Autodesk Inventor part; units mm, degrees
ref_plane "YZ Plane" through (0, 0, 0) normal (1, 0, 0) x (0, 1, 0)
ref_plane "XZ Plane" through (0, 0, 0) normal (0, 1, 0) x (-1, 0, 0)
ref_plane "XY Plane" through (0, 0, 0) normal (0, 0, 1) x (1, 0, 0)
sketch "Sketch1" plane through (0, 0, 0) normal (0, 1, 0) x (-1, 0, 0)
  line L0 (78.74, -3.175) -> (78.74, -41.275)
  line L1 (0, -41.275) -> (0, -3.175)
  line L2 (74.295, -4.445) -> (4.445, -4.445)
  line L3 (4.445, -4.445) -> (4.445, -40.005)
  line L4 (4.445, -40.005) -> (74.295, -40.005)
  line L5 (74.295, -40.005) -> (74.295, -4.445)
  line L6 (78.74, -3.175) -> (75.565, 0)
  line L7 (78.74, -41.275) -> (75.565, -44.45)
  line L8 (3.175, -44.45) -> (0, -41.275)
  line L9 (0, -3.175) -> (3.175, 0)
  line L10 (62.865, 0) -> (62.865, 12.7)
  line L11 (62.865, 12.7) -> (75.565, 12.7)
  line L12 (75.565, 12.7) -> (75.565, 0)
  line L13 (62.865, -44.45) -> (62.865, -57.15)
  line L14 (62.865, -57.15) -> (75.565, -57.15)
  line L15 (75.565, -57.15) -> (75.565, -44.45)
  line L16 (15.875, -44.45) -> (15.875, -57.15)
  line L17 (15.875, -57.15) -> (3.175, -57.15)
  line L18 (3.175, -57.15) -> (3.175, -44.45)
  line L19 (15.875, 0) -> (15.875, 12.7)
  line L20 (15.875, 12.7) -> (3.175, 12.7)
  line L21 (3.175, 12.7) -> (3.175, 0)
  line L22 (62.865, 0) -> (15.875, 0)
  line L23 (62.865, -44.45) -> (15.875, -44.45)
  circle A0 centre (69.215, 6.35) radius 2.54
  circle A1 centre (9.525, -50.8) radius 2.54
  circle A2 centre (9.525, 6.35) radius 2.54
  circle A3 centre (69.215, -50.8) radius 2.54
extrude "Extrusion1" add sketch "Sketch1" along normal blind 2.54
properties part number "Spark MAX Holder Bottom"
Check sheet for the modelled part. Datum: model origin and axes. Units: mm. A direction names the side the tool comes from. Give positions to 0.01 mm unless a question says otherwise; leave off trailing zeros. Write each loop counter-clockwise with the first axis right and the second up, starting at its lowest first coordinate (ties: lowest second). Pieces come first, ordered by that corner, then holes.
Item 1: Scan lines: L1, parallel to Z at x = -27.5, y = 0.9 (3 decimals); L2, parallel to X at y = 0.95, z = -15 (3 decimals); L3, parallel to Z at x = -6.5, y = 0.2 (3 decimals). Record each from-to range of solid material in increasing order.
Item 2: Cross-section at D-D (z = 6.35). Enter the section's corners in (x, y) (3 decimals), and give its area (3 significant figures).
Item 3: Cross-section at B-B (x = -13). Enter the section's corners in (y, z) (3 decimals).
Item 4: Cross-section at C-C (y = 1.05). Enter the section's corners in (x, z) (3 decimals), and give its area (3 significant figures).
Item 5: Draft check along Z on faces 5 (the face through (-7.509, 1.252, 7.896)), 6 (the face through (-75.565, 1, 6)), 7 (the face through (-40, 1, 0)). Enter one of: released by +Z, released by -Z, zero draft, split by the parting line, or undercut.
Item 6: Access from +Z, -Z, +X, -X, +Y, -Y to the whole of each face (thin tool, end or side, straight path). Record for faces 1 (the face through (-3.175, 1, -51)), 2 (the face through (-62.865, 1, 6)), 3 (the face through (-39, 1, -40.005)), 4 (the face through (-75.565, 1, -51)).
Item 7: Gauge pin test, flat ends, axial feed: pin 1 (0.8 mm diameter, centred on x = -29, y = 2, fed in from +Z); pin 2 (0.8 mm diameter, centred on y = 1.5, z = -48.5, fed in from +X) (3 decimals); pin 3 (4 mm diameter, centred on x = -9.525, z = -50.8, fed in from -Y); pin 4 (0.8 mm diameter, centred on x = -41.5, y = 1.5, fed in from -Z). Record the tip position at first contact, or that the pin passes through.
Item 8: Cross-section at A-A (z = -9). Enter the section's corners in (x, y) (3 decimals).
Report:
1. L1: z = -44.45 to -40.005, -4.445 to 0
1. L2: x = -78.74 to -74.295, -4.445 to 0
1. L3: z = -57.15 to -40.005, -4.445 to 12.7
2. outline: (-75.565, 0) - (-71.755, 0) - (-71.755, 2.54) - (-75.565, 2.54) - close; (-66.675, 0) - (-62.865, 0) - (-62.865, 2.54) - (-66.675, 2.54) - close; (-15.875, 0) - (-12.065, 0) - (-12.065, 2.54) - (-15.875, 2.54) - close; (-6.985, 0) - (-3.175, 0) - (-3.175, 2.54) - (-6.985, 2.54) - close
2. area: 38.7 mm2
3. outline: (0, -57.15) - (2.54, -57.15) - (2.54, -40.005) - (0, -40.005) - close; (0, -4.445) - (2.54, -4.445) - (2.54, 12.7) - (0, 12.7) - close
4. outline: (-78.74, -41.275) - (-75.565, -44.45) - (-75.565, -57.15) - (-62.865, -57.15) - (-62.865, -44.45) - (-15.875, -44.45) - (-15.875, -57.15) - (-3.175, -57.15) - (-3.175, -44.45) - (0, -41.275) - (0, -3.175) - (-3.175, 0) - (-3.175, 12.7) - (-15.875, 12.7) - (-15.875, 0) - (-62.865, 0) - (-62.865, 12.7) - (-75.565, 12.7) - (-75.565, 0) - (-78.74, -3.175) - close; hole (-74.295, -40.005) - (-4.445, -40.005) - (-4.445, -4.445) - (-74.295, -4.445) - close; hole circle Ø5.08 at (-69.215, -50.8); hole circle Ø5.08 at (-69.215, 6.35); hole circle Ø5.08 at (-9.525, -50.8); hole circle Ø5.08 at (-9.525, 6.35)
4. area: 1,560 mm2
5. face 5: undercut
5. face 6: zero draft
5. face 7: released by +Z
6. face 1: -Z, +X, +Y, -Y
6. face 2: +Z, +Y, -Y
6. face 3: +Y, -Y
6. face 4: -Z, -X, +Y, -Y
7. pin 1: stops at z = 0
7. pin 2: stops at x = -3.175
7. pin 3: passes through
7. pin 4: stops at z = -44.45
8. outline: (-78.74, 0) - (-74.295, 0) - (-74.295, 2.54) - (-78.74, 2.54) - close; (-4.445, 0) - (0, 0) - (0, 2.54) - (-4.445, 2.54) - close
